Could you check a few things on this model? Use its own coordinates, in mm. A direction names the side the tool comes from. Give positions to 0.01 mm unless a question says otherwise; leave off trailing zeros. Write each loop counter-clockwise with the first axis right and the second up, starting at its lowest first coordinate (ties: lowest second). Pieces come first, ordered by that corner, then holes. Notation, with made-up numbers: (40, -34) - (46, -34) arc R22 ccw to (46, -19) - close; hole circle Ø8 at (68.5, 85.5). An arc over 180 degrees is marked (long way). Answer in a Markdown table with one row per item.
from build123d import *

# Parameters (mm, degrees)
SKETCH_1_W                         = 320
SKETCH_1_H                         = 22
SM_BASE_FLANGE_1_DEPTH             = 2
SM_EDGE_FLANGE_1_STRIP_W           = 8.2
SM_EDGE_FLANGE_1_STRIP_H           = 2
SM_EDGE_FLANGE_1_STRIP_CUT_DEPTH   = 320
SM_EDGE_FLANGE_1_STRIP_2_W         = 8.2
SM_EDGE_FLANGE_1_STRIP_2_H         = 2
SM_EDGE_FLANGE_1_STRIP_CUT_2_DEPTH = 320
SM_EDGE_FLANGE_1_DEPTH             = 320
SM_EDGE_FLANGE_1_BEND_DEPTH        = 320
SM_START                           = -11
SM_EDGE_FLANGE_2_DEPTH             = 22
SM_EDGE_FLANGE_2_2_DEPTH           = 2.1
SM_START_2                         = 8.9
SM_EDGE_FLANGE_2_3_DEPTH           = 2.1
SM_START_3                         = -8.9
SM_EDGE_FLANGE_2_4_DEPTH           = 17.8
SKETCH_18_W                        = 9
SKETCH_18_H                        = 9
CUT_EXTRUDE_1_DEPTH                = 10
PATTERN_LINEAR_1_COUNT             = 20
PATTERN_LINEAR_1_PITCH             = 20
CUT_EXTRUDE_2_DEPTH                = 321.345126387
CUT_EXTRUDE_2_DEPTH_BACK           = 321.345126387
SKETCH_19_R                        = 0.75


# Read off the part's stored shape, not the designer's step: 边线-法兰2
# Sheet-metal steps are written as plain solids
with BuildPart() as part:
    # Sketch 1 → 基体-法兰1 (new body)
    with BuildSketch(Plane.XY):
        Rectangle(SKETCH_1_W, SKETCH_1_H)
    extrude(amount=-SM_BASE_FLANGE_1_DEPTH)

    # 边线-法兰1 strip (across the edge) → 边线-法兰1 strip cut (cut)
    with BuildSketch(Plane(origin=(160, -11, -2), x_dir=(0, 1, 0), z_dir=(-1, 0, 0))):
        with Locations((-2, -1)):
            Rectangle(SM_EDGE_FLANGE_1_STRIP_W, SM_EDGE_FLANGE_1_STRIP_H)
    extrude(amount=SM_EDGE_FLANGE_1_STRIP_CUT_DEPTH, mode=Mode.SUBTRACT)

    # 边线-法兰1 strip 2 (across the edge) → 边线-法兰1 strip cut 2 (cut)
    with BuildSketch(Plane(origin=(-160, 11, -2), x_dir=(0, -1, 0), z_dir=(1, 0, 0))):
        with Locations((-2, -1)):
            Rectangle(SM_EDGE_FLANGE_1_STRIP_2_W, SM_EDGE_FLANGE_1_STRIP_2_H)
    extrude(amount=SM_EDGE_FLANGE_1_STRIP_CUT_2_DEPTH, mode=Mode.SUBTRACT)

    # 边线-法兰1 section (across the edge) → 边线-法兰1 (add)
    with BuildSketch(Plane(origin=(160, -11, -2), x_dir=(0, 1, 0), z_dir=(-1, 0, 0))):
        with BuildLine():
            Line((0, 0.1), (0, 8))
            Line((0, 8), (2, 8))
            Line((2, 8), (2, 0.1))
            ThreePointArc((2, 0.1), (2.029289322, 0.029289322), (2.1, 0))
            Line((2.1, 0), (2.1, -2))
            ThreePointArc((2.1, -2), (0.61507576, -1.38492424), (0, 0.1))
        make_face()
    extrude(amount=SM_EDGE_FLANGE_1_DEPTH)

    # 边线-法兰1 section 2 (across the edge) → 边线-法兰1 bend (add)
    with BuildSketch(Plane(origin=(-160, 11, -2), x_dir=(0, -1, 0), z_dir=(1, 0, 0))):
        with BuildLine():
            Line((0, 0.1), (0, 8))
            Line((0, 8), (2, 8))
            Line((2, 8), (2, 0.1))
            ThreePointArc((2, 0.1), (2.029289322, 0.029289322), (2.1, 0))
            Line((2.1, 0), (2.1, -2))
            ThreePointArc((2.1, -2), (0.61507576, -1.38492424), (0, 0.1))
        make_face()
    extrude(amount=SM_EDGE_FLANGE_1_BEND_DEPTH)

    # 边线-法兰2 outline → 边线-法兰2 (cut)
    with BuildSketch(Plane(origin=(0, 0, 0), x_dir=(1, 0, 0), z_dir=(0, 1, 0)).offset(SM_START)):
        with BuildLine():
            Line((158, 2.1), (157.9, 2.1))
            Line((157.9, 2.1), (157.9, 2))
            ThreePointArc((157.9, 2), (157.970710678, 2.029289322), (158, 2.1))
        make_face()
        with BuildLine():
            ThreePointArc((160, 2.1), (159.38492424, 0.61507576), (157.9, 0))
            Line((157.9, 0), (160, 0))
            Line((160, 0), (160, 2.1))
        make_face()
        with BuildLine():
            ThreePointArc((-158, 2.1), (-157.970710678, 2.029289322), (-157.9, 2))
            Line((-157.9, 2), (-157.9, 2.1))
            Line((-157.9, 2.1), (-158, 2.1))
        make_face()
        with BuildLine():
            Line((-160, 0), (-157.9, 0))
            ThreePointArc((-157.9, 0), (-159.38492424, 0.61507576), (-160, 2.1))
            Line((-160, 2.1), (-160, 0))
        make_face()
    extrude(amount=SM_EDGE_FLANGE_2_DEPTH, mode=Mode.SUBTRACT)

    # Sm Edge Flange 2 2 outline → Sm Edge Flange 2 2 (cut)
    with BuildSketch(Plane(origin=(0, 0, 0), x_dir=(1, 0, 0), z_dir=(0, 1, 0)).offset(SM_START)):
        with BuildLine():
            Line((160, 2.1), (158, 2.1))
            ThreePointArc((158, 2.1), (157.970710678, 2.029289322), (157.9, 2))
            Line((157.9, 2), (157.9, 0))
            ThreePointArc((157.9, 0), (159.38492424, 0.61507576), (160, 2.1))
        make_face()
        with BuildLine():
            ThreePointArc((-160, 2.1), (-159.38492424, 0.61507576), (-157.9, 0))
            Line((-157.9, 0), (-157.9, 2))
            ThreePointArc((-157.9, 2), (-157.970710678, 2.029289322), (-158, 2.1))
            Line((-158, 2.1), (-160, 2.1))
        make_face()
    extrude(amount=SM_EDGE_FLANGE_2_2_DEPTH, mode=Mode.SUBTRACT)

    # Sm Edge Flange 2 3 outline → Sm Edge Flange 2 3 (cut)
    with BuildSketch(Plane(origin=(0, 0, 0), x_dir=(1, 0, 0), z_dir=(0, 1, 0)).offset(SM_START_2)):
        with BuildLine():
            Line((160, 2.1), (158, 2.1))
            ThreePointArc((158, 2.1), (157.970710678, 2.029289322), (157.9, 2))
            Line((157.9, 2), (157.9, 0))
            ThreePointArc((157.9, 0), (159.38492424, 0.61507576), (160, 2.1))
        make_face()
        with BuildLine():
            ThreePointArc((-160, 2.1), (-159.38492424, 0.61507576), (-157.9, 0))
            Line((-157.9, 0), (-157.9, 2))
            ThreePointArc((-157.9, 2), (-157.970710678, 2.029289322), (-158, 2.1))
            Line((-158, 2.1), (-160, 2.1))
        make_face()
    extrude(amount=SM_EDGE_FLANGE_2_3_DEPTH, mode=Mode.SUBTRACT)

    # Sm Edge Flange 2 4 outline → Sm Edge Flange 2 4 (add)
    with BuildSketch(Plane(origin=(0, 0, 0), x_dir=(1, 0, 0), z_dir=(0, 1, 0)).offset(SM_START_3)):
        with BuildLine():
            Line((158, 10), (158, 2.1))
            ThreePointArc((158, 2.1), (157.970710678, 2.029289322), (157.9, 2))
            Line((157.9, 2), (159.997617696, 2))
            ThreePointArc((159.997617696, 2), (159.99940434, 2.049985814), (160, 2.1))
            Line((160, 2.1), (160, 10))
            Line((160, 10), (158, 10))
        make_face()
        with BuildLine():
            Line((-159.997617696, 2), (-157.9, 2))
            ThreePointArc((-157.9, 2), (-157.970710678, 2.029289322), (-158, 2.1))
            Line((-158, 2.1), (-158, 10))
            Line((-158, 10), (-160, 10))
            Line((-160, 10), (-160, 2.1))
            ThreePointArc((-160, 2.1), (-159.99940434, 2.049985814), (-159.997617696, 2))
        make_face()
    extrude(amount=SM_EDGE_FLANGE_2_4_DEPTH)

    # 草图18 → 切除-拉伸1 (cut)
    with BuildSketch(Plane.XY):
        with Locations((-150, 1)):
            Rectangle(SKETCH_18_W, SKETCH_18_H)
    cut_extrude_1 = extrude(amount=-CUT_EXTRUDE_1_DEPTH, mode=Mode.SUBTRACT)

    # 阵列(线性)1: 切除-拉伸1 ×20
    with Locations(*[(i * PATTERN_LINEAR_1_PITCH, 0, 0) for i in range(1, PATTERN_LINEAR_1_COUNT)]):
        add(cut_extrude_1, mode=Mode.SUBTRACT)

    # 草图19 → 切除-拉伸2 (cut, two sides: drawn at the far end of the back side and taken through both)
    with BuildSketch(Plane(origin=(160, 0, 0), x_dir=(0, 0, -1), z_dir=(1, 0, 0)).offset(-CUT_EXTRUDE_2_DEPTH_BACK)):
        with Locations(Location((7, 0, 0), (0, 0, 180))):
            Circle(SKETCH_19_R)
    extrude(amount=CUT_EXTRUDE_2_DEPTH + CUT_EXTRUDE_2_DEPTH_BACK, mode=Mode.SUBTRACT)


solid = part.part
1) On a 3-axis mill with a long thin cutter (end or side, diameter ignored), from which of +Z, -Z, +X, -X, +Y, -Y can I reach the whole of each face in a straight line? I mean faces 5 (the face through (-158, 0, -6)), 6 (the face through (-160, 0, -6)). Say none if no direction works.
Check values:
| item | result |
|---|---|
| face 5 | -Z |
| face 6 | +Z, -Z, -X, +Y, -Y |
2) If I drill on line 1 (X direction, y = 6.75, z = -8.75); line 2 (Y direction, x = -54, z = -5.75); line 3 (Z direction, x = -29, y = -8.75), over which ranges is the centre line in solid material (lowest first)?
Check values:
| item | result |
|---|---|
| line 1 | x = -160 to -158, 158 to 160 |
| line 2 | y = -11 to -9, 9 to 11 |
| line 3 | z = -2 to 0 |
3) Will these pins go through, and if not, where does the flat tip stop? P1, Ø0.6, axis at y = -1, z = -1.5, coming from the +X side; P2, Ø5, axis at x = 14, y = 5.5, coming from the -Z side; P3, Ø1, axis at y = 1.5, z = -1, coming from the -X side.
Check values:
| item | result |
|---|---|
| P1 | stops at x = 159.98 |
| P2 | stops at z = -2 |
| P3 | stops at x = -159.91 |
4) Imagine slicing it at B-B (x = 128.5). List the corners of the cut face in (y, z) for me.
Check values:
| item | result |
|---|---|
| outline | (-11, -10) - (-9, -10) - (-9, -2.1) arc R0.1 cw to (-8.9, -2) - (-3.5, -2) - (-3.5, 0) - (-8.9, 0) arc R2.1 ccw to (-11, -2.1) - close; (5.5, -2) - (8.9, -2) arc R0.1 cw to (9, -2.1) - (9, -10) - (11, -10) - (11, -2.1) arc R2.1 ccw to (8.9, 0) - (5.5, 0) - close |
5) Imagine slicing it at A-A (z = -3.75). List the corners of the cut face in (x, y) for me, then the cut area to 3 significant figures.
Check values:
| item | result |
|---|---|
| outline | (-160, -11) - (160, -11) - (160, -9) - (-160, -9) - close; (-160, -8.9) - (-158, -8.9) - (-158, 8.9) - (-160, 8.9) - close; (-160, 9) - (160, 9) - (160, 11) - (-160, 11) - close; (158, -8.9) - (160, -8.9) - (160, 8.9) - (158, 8.9) - close |
| area | 1,350 mm2 |
6) We'd pull the mould along Y, two halves only. Please class faces 1 (the face through (-2, 11, -6)), 2 (the face through (160, 0, -6)), 3 (the face through (-2, 9, -6)), 4 (the face through (2, -11, -6)): +Y half, -Y half, draft (parallel to the pull), parting line (faces both ways), or undercut.
Check values:
| item | result |
|---|---|
| face 1 | +Y half |
| face 2 | draft |
| face 3 | undercut |
| face 4 | -Y half |
